Input: part model. Units: mm. Frame: model coordinates. A direction names the side the tool comes from. Coordinates: 2 decimals unless noted, no trailing zeros. Loops run counter-clockwise (first coordinate to the right, second up) from the corner with the lowest first, then second, coordinate; pieces in that order, holes last. Notation, with made-up numbers: (86.5, 32) -> (122.5, 32) arc R31 cw to (122.5, 56) -> close; hole circle Ø8 at (84.25, 51.25). An arc over 180 degrees is marked (long way). Put each result on its own line as item: value. Start each with the question number.
1) Set-up query: faces 4 (the flat face through (4.75, 0, 2)), 5 (the cylindrical face through (-0.596, 2.685, 10.465)), 6 (the flat face through (0, 0, 13)). Return all of +Z, -Z, +X, -X, +Y, -Y with unobstructed straight access to the full face (end or side cutting, diameter ignored); none if empty.
2) Cut plane C-C (z = 5). Return the cut outline in (x, y).
3) Cut plane A-A (y = 0). Return the cut outline in (x, z), plus the area to 4 significant figures.
4) Cut plane B-B (x = 0). Return the cut outline in (y, z), plus the area to 4 significant figures.
5) Material intervals for L1, parallel to X at y = 1.5, z = 6.5; L2, parallel to Z at x = 2, y = 8.25; L3, parallel to Y at x = 7.5, z = 5.9, sorted ascending.
6) Pull-direction query (X, two-part tool) for faces 1 (the flat face through (8.8, -1.4, 4)), 2 (the cylindrical face through (11.923, -3.755, 4.958)), 3 (the flat face through (0, 3, 8)); classes: pulls with the +X half, pulls with the -X half, needs draft (parallel to the pull), parting line crosses it, or undercut.
7) Contact query for flat-ended pins moving along their axis: P1, Ø1.6, axis at x = 6.5, y = -1, coming from the -Z side; P2, Ø1, axis at x = 9.5, z = 5, coming from the +Y side; P3, Ø4, axis at y = 9, z = 7.5, coming from the +X side. Output: stop coordinate, or through.
Autodesk Inventor part; units mm, degrees
ref_plane "YZ Plane" through (0, 0, 0) normal (1, 0, 0) x (0, 1, 0)
ref_plane "XZ Plane" through (0, 0, 0) normal (0, 1, 0) x (-1, 0, 0)
ref_plane "XY Plane" through (0, 0, 0) normal (0, 0, 1) x (1, 0, 0)
sketch "Sketch1" plane through (0, 0, 0) normal (0, 0, 1) x (1, 0, 0)
  circle A0 centre (0, 0) radius 12.5
  dimension "d0" = 25
extrude "Extrusion1" add sketch "Sketch1" along normal blind 8
sketch "Sketch2" plane through (0, 0, 8) normal (0, 0, 1) x (1, 0, 0)
  circle A0 centre (0, 0) radius 12.5
  circle A1 centre (0, 0) radius 2.75
  dimension "d4" = 5.5
extrude "Extrusion2" add sketch "Sketch2" along normal blind 5 contours A1
sketch "Sketch3" plane through (0, 0, 8) normal (0, 0, 1) x (1, 0, 0)
  circle A0 centre (0, 0) radius 2.75
  circle A1 centre (-7.5, 0) radius 1.75
  circle A2 centre (7.5, 0) radius 1.75
  dimension "d8" = 7.5
  dimension "d9" = 7.5
  dimension "d10" = 3.5
extrude "Extrusion3" cut sketch "Sketch3" against normal through all contours A1 | A2
sketch "Sketch4" plane through (0, 0, 0) normal (0, 0, -1) x (-1, 0, 0)
  circle A0 centre (7.5, 0) radius 1.75
  circle A1 centre (-7.5, 0) radius 1.75
  line L0 (-7.5, 3.1754) -> (-4.75, 1.5877)
  line L1 (-4.75, 1.5877) -> (-4.75, -1.5877)
  line L2 (-4.75, -1.5877) -> (-7.5, -3.1754)
  line L3 (-7.5, -3.1754) -> (-10.25, -1.5877)
  line L4 (-10.25, -1.5877) -> (-10.25, 1.5877)
  line L5 (-10.25, 1.5877) -> (-7.5, 3.1754)
  line L6 (7.5, 3.1754) -> (10.25, 1.5877)
  line L7 (10.25, 1.5877) -> (10.25, -1.5877)
  line L8 (10.25, -1.5877) -> (7.5, -3.1754)
  line L9 (7.5, -3.1754) -> (4.75, -1.5877)
  line L10 (4.75, -1.5877) -> (4.75, 1.5877)
  line L11 (4.75, 1.5877) -> (7.5, 3.1754)
  dimension "d13" = 5.5
extrude "Extrusion4" cut sketch "Sketch4" against normal blind 4
chamfer "Chamfer2" distance 2 angle 45 1 edges at (-12.5, 0, 0)
properties part number "stopper"
Results found:
1. face 4: -Z
1. face 5: +Z
1. face 6: +Z, +X, -X, +Y, -Y
2. outline: circle Ø25 at (0, 0); hole circle Ø3.5 at (-7.5, 0); hole circle Ø3.5 at (7.5, 0)
3. outline: (-12.5, 2) -> (-10.5, 0) -> (-10.25, 0) -> (-10.25, 4) -> (-9.25, 4) -> (-9.25, 8) -> (-12.5, 8) -> close; (-5.75, 4) -> (-4.75, 4) -> (-4.75, 0) -> (4.75, 0) -> (4.75, 4) -> (5.75, 4) -> (5.75, 8) -> (2.75, 8) -> (2.75, 13) -> (-2.75, 13) -> (-2.75, 8) -> (-5.75, 8) -> close; (9.25, 4) -> (10.25, 4) -> (10.25, 0) -> (10.5, 0) -> (12.5, 2) -> (12.5, 8) -> (9.25, 8) -> close
3. area: 151.5 mm2
4. outline: (-12.5, 2) -> (-10.5, 0) -> (10.5, 0) -> (12.5, 2) -> (12.5, 8) -> (2.75, 8) -> (2.75, 13) -> (-2.75, 13) -> (-2.75, 8) -> (-12.5, 8) -> close
4. area: 223.5 mm2
5. L1: x = -12.41 to -8.4, -6.6 to 6.6, 8.4 to 12.41
5. L2: z = 0 to 8
5. L3: y = -10 to -1.75, 1.75 to 10
6. face 1: undercut
6. face 2: parting line crosses it
6. face 3: needs draft
7. P1: stops at z = 4
7. P2: stops at y = 8.67
7. P3: stops at x = 10.36
